Autodesk Inventor part; units mm, degrees
ref_plane "YZ Plane" through (0, 0, 0) normal (1, 0, 0) x (0, 1, 0)
ref_plane "XZ Plane" through (0, 0, 0) normal (0, 1, 0) x (-1, 0, 0)
ref_plane "XY Plane" through (0, 0, 0) normal (0, 0, 1) x (1, 0, 0)
sketch "Sketch1" plane through (0, 0, 0) normal (0, 0, 1) x (1, 0, 0)
  circle A0 centre (0, 0) radius 15
  circle A1 centre (0, 0) radius 16.4
  line L0 (-7.15, -14.7593) -> (-7.15, -30.5704)
  line L1 (-7.15, -30.5704) -> (-5.15, -30.5704)
  line L2 (-5.15, -30.5704) -> (-5.15, -15.5704)
  line L3 (5.15, -15.5704) -> (5.15, -30.5704)
  line L4 (5.15, -30.5704) -> (7.15, -30.5704)
  line L5 (7.15, -30.5704) -> (7.15, -14.7593)
  dimension "d0" = 1.4
  dimension "d1" = 30
  dimension "d2" = 2
  dimension "d3" = 10.3
  dimension "d4" = 15
extrude "Extrusion1" add sketch "Sketch1" along normal blind 30 contours A1
extrude "Extrusion3" add sketch "Sketch1" along normal blind 24 contours A1 L2 L1 L0 | L5 L4 L3 A1
sketch "Sketch2" plane through (-7.15, -30.5704, 0) normal (-1, 0, 0) x (0, 0, 1)
  circle A0 centre (3.6261, 4) radius 1.75
  circle A1 centre (19.6261, 4) radius 1.75
  line L0 (0, 0) -> (24, 0)
  point P0 (0, 30.5704)
  dimension "d7" = 3.5
  dimension "d8" = 3.5
  dimension "d9" = 16
  dimension "d15" = 4
extrude "Extrusion2" cut sketch "Sketch2" against normal through all
sketch "Sketch3" plane through (0, 0, 0) normal (0, 1, 0) x (-1, 0, 0)
  circle A0 centre (0, 8) radius 0.9
  circle A1 centre (0, 20) radius 0.9
  line L0 (15, 0) -> (-15, 0)
  point P0 (0, 0)
  point P1 (0, 0)
  dimension "d16" = 1.8
  dimension "d18" = 12
  dimension "d19" = 8
extrude "Extrusion4" cut sketch "Sketch3" along normal through all
properties part number "Pok Default Pitch Motor Mount" material "ABS Plastic"
Design review of the part built by this model. Coordinates are the model's own, in mm. A direction names the side the tool comes from. Give positions to 0.01 mm unless a question says otherwise; leave off trailing zeros. Order: outer loops, then holes, each group sorted by start corner. A loop starts at its lowest first (then second) coordinate and runs counter-clockwise, first axis right, second up. Notation, with made-up numbers: (70, 87.25) - (97, 87.25) arc R23 cw to (97, 99.25) - close; hole circle Ø8 at (48, 33.5). An arc over 180 degrees is marked (long way). Write item = value, one per line. Start each with the question number.
Q1. We need section B-B on y = 0. State the section outline as (x, z) points, plus the area to 3 significant figures.
Q2. Clearance check with flat-ended pins moving along their axes: pin 1 Ø5 at (x, z) = (10, 21.5) entering from +Y; pin 2 Ø3 at (y, z) = (-26.57, 19.63) entering from +X; pin 3 Ø3 at (y, z) = (-9.5, 25.5) entering from -X; pin 4 Ø2 at (x, z) = (-9, 12.5) entering from -Y. State where each tip first meets the part, or that it passes through.
Q3. Tool access review of faces 4 (the face through (-5.15, -23, 12)), 5 (the face through (0.12, 15.68, 19.11)), 6 (the face through (-7.15, -23, 12)): name each direction out of +Z, -Z, +X, -X, +Y, -Y from which nothing blocks a thin tool from reaching the whole face with its end or side.
Q4. Mouldability with a two-part tool opening along X and no side actions: class faces 1 (the face through (-0.48, 15.68, 7.24)), 2 (the face through (-6.164, -27.241, 21.243)), 3 (the face through (7.15, -23, 12)) as released by +X, released by -X, zero draft, split by the parting line, or undercut.
Q5. We need section D-D on x = -4.5. State the section outline as (y, z) points.
Q6. To check wall thickness, follow L1, parallel to Y at x = -7, z = 20; L2, parallel to Z at x = 0, y = 15.45; L3, parallel to Y at x = -1, z = 9.5. State the ranges of each line that lie inside material, in increasing order. Write a range as from..to.
Q7. We need section C-C on x = 0. State the section outline as (y, z) points.
Q8. We need section A-A on z = 4. State the section outline as (x, y) points, plus the area to 3 significant figures.
Working result:
q1.outline = (-16.4, 0) - (-15, 0) - (-15, 30) - (-16.4, 30) - close; (15, 0) - (16.4, 0) - (16.4, 30) - (15, 30) - close
q1.area = 84.0 mm²
q2.pin_1 = 14.58
q2.pin_2 = through
q2.pin_3 = -14.32
q2.pin_4 = -14.32
q3.face_4 = +Z, -Z, -Y
q3.face_5 = +Y
q3.face_6 = +Z, -Z, -X, -Y
q4.face_1 = undercut
q4.face_2 = zero draft
q4.face_3 = released by +X
q5.outline = (-15.77, 0) - (-14.31, 0) - (-14.31, 30) - (-15.77, 30) - close; (14.31, 0) - (15.77, 0) - (15.77, 30) - (14.31, 30) - close
q6.L1 = -30.57..-28.28, -24.86..-13.27, 13.27..14.83
q6.L2 = 0..7.1, 8.9..19.1, 20.9..30
q6.L3 = -16.37..-14.97, 14.97..16.37
q7.outline = (-16.4, 0) - (-15, 0) - (-15, 30) - (-16.4, 30) - close; (15, 0) - (16.4, 0) - (16.4, 7.1) - (15, 7.1) - close; (15, 8.9) - (16.4, 8.9) - (16.4, 19.1) - (15, 19.1) - close; (15, 20.9) - (16.4, 20.9) - (16.4, 30) - (15, 30) - close
q8.outline = (-7.15, -30.57) - (-5.15, -30.57) - (-5.15, -28.28) - (-7.15, -28.28) - close; (-7.15, -24.86) - (-5.15, -24.86) - (-5.15, -15.57) arc R16.4 ccw to (5.15, -15.57) - (5.15, -24.86) - (7.15, -24.86) - (7.15, -14.76) arc R16.4 ccw (long way) to (-7.15, -14.76) - close; (5.15, -30.57) - (7.15, -30.57) - (7.15, -28.28) - (5.15, -28.28) - close; hole circle Ø30 at (0, 0)
q8.area = 186 mm²
